Geometry check sheet. Reference: the model listing, model coordinates, mm. Give positions to 0.01 mm unless a question says otherwise; leave off trailing zeros. Write each loop counter-clockwise with the first axis right and the second up, starting at its lowest first coordinate (ties: lowest second). Pieces come first, ordered by that corner, then holes. Notation, with made-up numbers: M 15.5,54.5 L 37.5,54.5 A25 cw 37.5,89.5 Z; hole C -40,17 d6. An arc over 180 degrees is marked long. One line per item, written item: value. Start each with the question number.
1. Cross-section at B-B on z = 555. Record the cut outline in (x, y), then the cut area to 3 significant figures.
2. Gauge pin test, flat ends, axial feed: pin 1 (2 mm diameter, centred on x = -323.5, z = 492.5, fed in from -Y); pin 2 (0.5 mm diameter, centred on y = 0.5, z = 558, fed in from +X); pin 3 (0.5 mm diameter, centred on y = 0.5, z = -73.5, fed in from -X). Record the tip position at first contact, or that the pin passes through.
3. Scan lines: line 1 (X direction, y = 0.75, z = 547); line 2 (Z direction, x = -211.5, y = 0.9); line 3 (X direction, y = 0.05, z = 119.5). Record each from-to range of solid material in increasing order.
4. Cross-section at C-C on x = -458. Record the cut outline in (y, z), then the cut area to 3 significant figures.
5. Cross-section at A-A on y = 0.4. Record the cut outline in (x, z).
from build123d import *

# Parameters (mm, degrees)
SKETCH1_W           = 148
SKETCH1_H           = 106
SKETCH1_W_2         = 1088
SKETCH1_H_2         = 20
BOSS_EXTRUDE1_DEPTH = 1


with BuildPart() as part:
    # Sketch1 → Boss-Extrude1 (new body)
    with BuildSketch(Plane(origin=(0, 0, 0), x_dir=(1, 0, 0), z_dir=(0, 1, 0))):
        Polygon((-284.309741609, -519.73309486), (294.379685644, -375.483559699), (185.690258391, 60.9163871), align=None)
        with Locations((-358.309741609, -572.73309486)):
            Rectangle(SKETCH1_W, SKETCH1_H)
        Polygon((294.379685644, -375.483559699), (313.786824034, -370.650033087), (205.097396781, 65.749913711), (185.690258391, 60.9163871), align=None)
        with Locations((-358.309741609, 70.9163871)):
            Rectangle(SKETCH1_W_2, SKETCH1_H_2)
        Polygon((-902.309741609, 60.9163871), (-921.71688, 65.749913711), (-1030.406307253, -370.650033087), (-1010.999168863, -375.483559699), align=None)
        Polygon((-1010.999168863, -375.483559699), (-902.309741609, 60.9163871), (-432.309741609, -519.73309486), align=None)
        Polygon((185.690258391, 60.9163871), (-284.309741609, -519.73309486), (-432.309741609, -519.73309486), (-902.309741609, 60.9163871), align=None)
    extrude(amount=BOSS_EXTRUDE1_DEPTH)


solid = part.part
Report:
1. outline: M -432.31,0 L -284.31,0 L -284.31,1 L -432.31,1 Z
1. area: 148 mm^2
2. pin 1: stops at y = 0
2. pin 2: stops at x = -284.31
2. pin 3: stops at x = -902.31
3. line 1: x = -432.31 to -284.31
3. line 2: z = -80.92 to 501.58
3. line 3: x = -967.86 to 251.24
4. outline: M 0,-80.92 L 1,-80.92 L 1,513.33 L 0,513.33 Z
4. area: 594 mm^2
5. outline: M -1030.41,370.65 L -921.72,-65.75 L -902.31,-60.92 L -902.31,-80.92 L 185.69,-80.92 L 185.69,-60.92 L 205.1,-65.75 L 313.79,370.65 L 294.38,375.48 L -284.31,519.73 L -284.31,625.73 L -432.31,625.73 L -432.31,519.73 L -1011,375.48 Z
